Could you check a few things on this drawing? It's one solid part, dimensions in mm from its lowest x, y, z. Give positions to 0.01 mm unless a question says otherwise; leave off trailing zeros. Loops run counter-clockwise (first coordinate to the right, second up) from the corner with the lowest first, then second, coordinate; pieces in that order, holes last.
Q1. Suppose I cut it at C-C (x = 44). List the corners of the cut face in (y, z) for me, and give its area (3 significant figures).
Q2. I need wall thicknesses on probe 1 along X at (y, z) = (150, 6.25); probe 2 along X at (y, z) = (129, 12); probe 3 along Y at (x, z) = (46, 9). Which ranges of each line are inside material? Lowest first, please.
Q3. I'm going to push flat-ended pins straight in: P1, Ø6, axis at y = 40, z = 4, coming from the -X side; P2, Ø2, axis at x = 10, z = 7.5, coming from the -Y side. Where does each tip first touch, or does it pass through?
Q4. Suppose I cut it at A-A (y = 92). List the corners of the cut face in (x, z) for me.
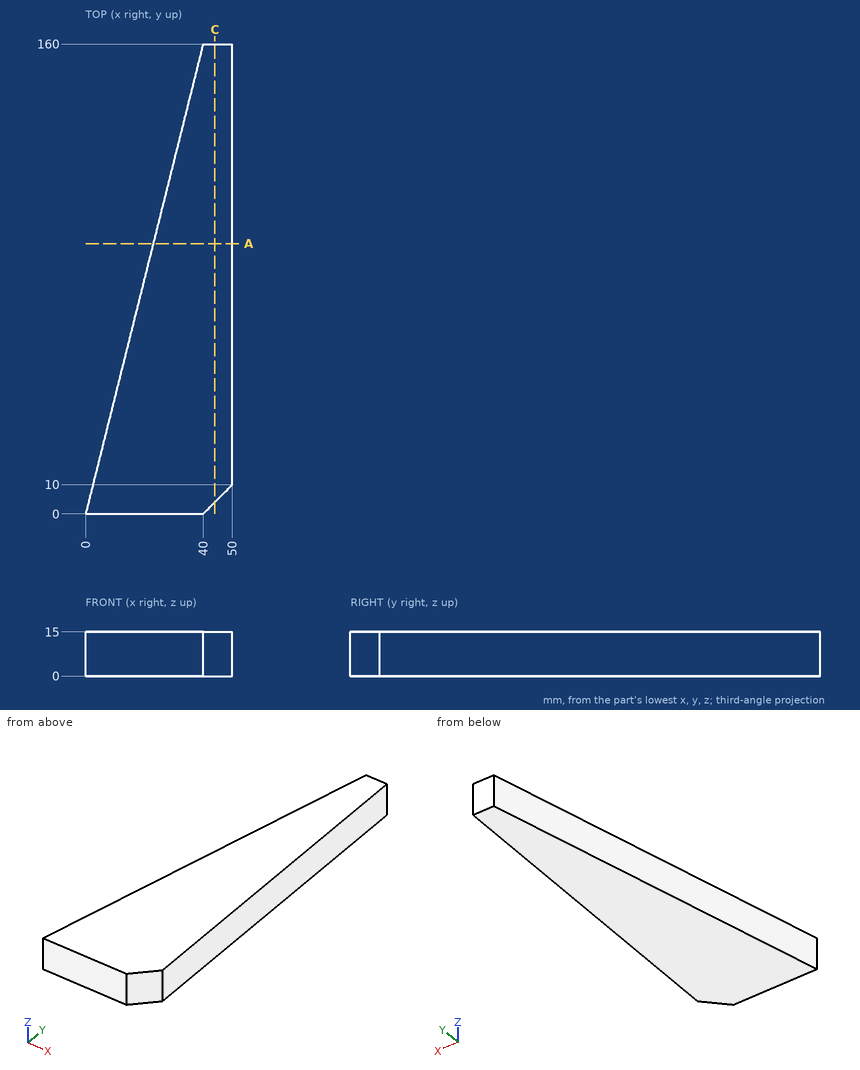
Solutions:
1. outline: (4, 0) - (160, 0) - (160, 15) - (4, 15) - close
1. area: 2,340 mm2
2. probe 1: x = 37.5 to 50
2. probe 2: x = 32.25 to 50
2. probe 3: y = 6 to 160
3. P1: stops at x = 9.25
3. P2: stops at y = 0
4. outline: (23, 0) - (50, 0) - (50, 15) - (23, 15) - close
